Read the model definition and answer for the solid it produces. Units are mm, in the model's axes. A direction names the side the tool comes from. Coordinates: 2 decimals unless noted, no trailing zeros. Write each loop counter-clockwise with the first axis right and the second up, starting at its lowest first coordinate (ties: lowest second). Pieces come first, ordered by that corner, then holes. Notation, with made-up numbers: (11.5, 12) -> (23.5, 12) arc R23 cw to (23.5, 41) -> close; hole circle Ø11 at (12.5, 23.5). An arc over 180 degrees is marked (long way). Answer as a JSON object with one key per item and string values. Group by question number.
(1) Which of the six approach directions +Z, -Z, +X, -X, +Y, -Y give full straight-line access (tool end or side, diameter ignored) to faces 1 (the face through (-40.055, -19, 3)), 2 (the face through (-6, 5.535, 3)), 3 (the face through (-38, -7.347, 3)), 4 (the face through (-14, -13.385, 3))?
(2) For a pull along X with two mould halves and no side action, classify faces 5 (the face through (-23, -24.858, 3)), 6 (the face through (-39, -20.028, 3)), 7 (the face through (-20.33, -25, 3)) as +X half, -X half, draft (parallel to the pull), parting line (faces both ways), or undercut.
(3) Flat-ended cylindrical pins translate along their axes: P1, Ø1.4, axis at x = -11.5, z = 2.5, coming from the -Y side; P2, Ø2.5, axis at x = -47, z = 4, coming from the +Y side; P3, Ø0.7, axis at x = -45, z = 2.5, coming from the +Y side. Find the tip coordinate at first contact, or state that the pin passes through.
(4) Find section B-B (x = -16.5). Give the vertices of the cut face in (y, z).
(5) Find section D-D (y = 10.5). Give the vertices of the cut face in (x, z), then the cut area to 3 significant figures.
(6) Find section C-C (y = -6). Give the vertices of the cut face in (x, z), then the cut area to 3 significant figures.
(7) Find section A-A (y = 16.5). Give the vertices of the cut face in (x, z).
(8) Straight lines are drawn through the part: L1, parallel to Y at x = -8, z = 3; L2, parallel to X at y = -5, z = 5.25; L3, parallel to Y at x = -20, z = 2. For each, find the intervals that lie inside material, in ascending order.
from build123d import *

# Parameters (mm, degrees)
F0_W     = 3.824378
F0_H     = 3.421813
F1_DEPTH = 6.35


with BuildPart() as f1:
    # F0 (on Top) → F1 (new body)
    with BuildSketch(Plane.XY):
        Polygon((0, 22.241773), (-19.725736, 22.241773), (-19.524453, 19.021247), (-22.141133, 19.021247), (-22.141133, 2.516038), (-24.556529, 2.516038), (-24.556529, 0), (-28.380906, 0), (-28.380906, -1.912189), (-32.60785, -1.912189), (-32.60785, -5.132717), (-35.224527, -5.132717), (-35.224527, -7.34683), (-41.061737, -7.34683), (-41.061737, -5.132717), (-43.678414, -5.132717), (-43.678414, -2.717321), (-45.892529, -2.717321), (-45.892529, 3.32117), (-48.106641, 3.32117), (-48.106641, -11.573775), (-45.288678, -11.573775), (-45.288678, -14.391736), (-42.470716, -14.391736), (-42.470716, -17.612264), (-40.05532, -17.612264), (-40.05532, -20.027662), (-38.042489, -20.027662), (-38.042489, -22.845622), (-35.627093, -22.845622), (-35.627093, -32.708492), (-30.796302, -32.708492), (-30.796302, -30.494377), (-32.60785, -30.494377), (-32.60785, -27.676415), (-29.99117, -27.676415), (-29.99117, -24.858454), (-27.777057, -24.858454), (-27.777057, -22.04049), (-24.153963, -22.04049), (-24.153963, -24.858454), (-22.342416, -24.858454), (-22.342416, -32.708492), (-17.712906, -32.708492), (-17.712906, -30.69566), (-20.329585, -30.69566), (-20.329585, -19.826377), (-17.511621, -19.826377), (-17.511621, -17.209699), (-15.29751, -17.209699), (-15.29751, -13.38532), (-12.479547, -13.38532), (-12.479547, -4.528868), (-9.661585, -4.528868), (-9.661585, -6.944264), (-7.447471, -6.944264), (-7.447471, -2.717321), (-12.479547, -2.717321), (-12.479547, 3.32117), (-2.616679, 3.32117), (-2.616679, 5.535283), (-10.064151, 5.535283), (-10.064151, 8.151962), (2.616679, 8.151962), (2.616679, 19.021247), (0, 19.021247), align=None)
        with Locations((-15.800717, 17.31034)):
            Rectangle(F0_W, F0_H, mode=Mode.SUBTRACT)
    extrude(amount=F1_DEPTH)


solid = f1.part
Results below:
{
 "1": {"face 1": "+Z, -Z, -X, -Y", "face 2": "+Z, -Z, +X", "face 3": "+Z, -Z, +Y", "face 4": "+Z, -Z, +X, -Y"},
 "2": {"face 5": "undercut", "face 6": "draft", "face 7": "+X half"},
 "3": {"P1": "stops at y = -4.53", "P2": "stops at y = 3.32", "P3": "stops at y = -2.72"},
 "4": {"outline": "(-17.21, 0) -> (15.6, 0) -> (15.6, 6.35) -> (-17.21, 6.35) -> close; (19.02, 0) -> (22.24, 0) -> (22.24, 6.35) -> (19.02, 6.35) -> close"},
 "5": {"outline": "(-22.14, 0) -> (2.62, 0) -> (2.62, 6.35) -> (-22.14, 6.35) -> close", "area": "157 mm2"},
 "6": {"outline": "(-48.11, 0) -> (-41.06, 0) -> (-41.06, 6.35) -> (-48.11, 6.35) -> close; (-35.22, 0) -> (-12.48, 0) -> (-12.48, 6.35) -> (-35.22, 6.35) -> close; (-9.66, 0) -> (-7.45, 0) -> (-7.45, 6.35) -> (-9.66, 6.35) -> close", "area": "203 mm2"},
 "7": {"outline": "(-22.14, 0) -> (-17.71, 0) -> (-17.71, 6.35) -> (-22.14, 6.35) -> close; (-13.89, 0) -> (2.62, 0) -> (2.62, 6.35) -> (-13.89, 6.35) -> close"},
 "8": {"L1": "y = -6.94 to -2.72, 3.32 to 5.54, 8.15 to 22.24", "L2": "x = -48.11 to -43.68, -32.61 to -12.48, -9.66 to -7.45", "L3": "y = -32.71 to -30.7, -19.83 to 19.02"}
}
